Geometry: final body of the model. Coordinates: model frame, mm. A direction names the side the tool comes from. Give positions to 0.01 mm unless a question says otherwise; leave off trailing zeros. Order: outer loops, then holes, each group sorted by start corner. A loop starts at its lowest first (then second) coordinate and runs counter-clockwise, first axis right, second up. Notation, with made-up numbers: (-24, 37) - (-18, 37) arc R34 ccw to (-18, 75) - close; hole circle Ø2 at (-38.75, 55). An arc over 180 degrees is marked (long way). Use one line per item in the form item = value.
from build123d import *

# Parameters (mm, degrees)
ESQUISSE1_W                                    = 138
ESQUISSE1_H                                    = 77
BOSS_EXTRU_1_DEPTH                             = 3
ESQUISSE2_W                                    = 15
ESQUISSE2_H                                    = 77
BOSS_EXTRU_2_DEPTH                             = 30
CONG_1_R                                       = 13.85
ESQUISSE3_W                                    = 138
ESQUISSE3_H                                    = 33
BOSS_EXTRU_3_DEPTH                             = 5
ENL_V_MAT_EXTRU_13_REACH                       = 168.439
ESQUISSE26_W                                   = 15
ESQUISSE26_H                                   = 33
CONG_5_R                                       = 1
ESQUISSE33_W                                   = 11
ESQUISSE33_H                                   = 83.5
ENL_V_MAT_EXTRU_15_DEPTH                       = 28
ESQUISSE34_W                                   = 3.5
ESQUISSE34_H                                   = 33
BOSS_EXTRU_8_DEPTH                             = 25
BOSS_EXTRU_11_DEPTH                            = 33
ESQUISSE35_R                                   = 1
ESQUISSE35_W                                   = 23
ESQUISSE35_H                                   = 14.5
ENL_V_MAT_EXTRU_16_DEPTH                       = 7
ESQUISSE36_W                                   = 7
ESQUISSE36_H                                   = 11.75
ENL_V_MAT_EXTRU_17_DEPTH                       = 2
ESQUISSE44_R                                   = 6
ENL_V_MAT_EXTRU_19_DEPTH                       = 3.5
D_GAGEMENT_M124_D                              = 13.5
D_GAGEMENT_M124_DEPTH                          = 3.5
D_GAGEMENT_M124_TIP                            = 4.055809178
ESQUISSE48_R                                   = 1.5
ENL_V_MAT_EXTRU_20_DEPTH                       = 5
FRAISAGE_POUR_VIS_T_TE_FRAIS_E_M32_D           = 3.4
FRAISAGE_POUR_VIS_T_TE_FRAIS_E_M32_DEPTH       = 5
FRAISAGE_POUR_VIS_T_TE_FRAIS_E_M32_CSINK_D     = 6.3
FRAISAGE_POUR_VIS_T_TE_FRAIS_E_M32_CSINK_ANGLE = 90
FRAISAGE_POUR_VIS_T_TE_FRAIS_E_M32_TIP         = 1.021463052
ESQUISSE52_W                                   = 10
ESQUISSE52_H                                   = 10
BOSS_EXTRU_12_DEPTH                            = 7
ESQUISSE53_R                                   = 1.5
ENL_V_MAT_EXTRU_21_DEPTH                       = 7
CONG_8_R                                       = 5


with BuildPart() as part:
    # Esquisse1 → Boss.-Extru.1 (new body)
    with BuildSketch(Plane(origin=(0, 0, 0), x_dir=(1, 0, 0), z_dir=(0, 1, 0))):
        with Locations((69, 38.5)):
            Rectangle(ESQUISSE1_W, ESQUISSE1_H)
    extrude(amount=BOSS_EXTRU_1_DEPTH)

    # Esquisse2 → Boss.-Extru.2 (add)
    with BuildSketch(Plane(origin=(0, 3, 0), x_dir=(1, 0, 0), z_dir=(0, 1, 0))):
        with Locations((130.5, 38.5)):
            Rectangle(ESQUISSE2_W, ESQUISSE2_H)
    extrude(amount=BOSS_EXTRU_2_DEPTH)

    # Congé1
    cong_1_edges = [part.edges().sort_by_distance(p)[0] for p in [
        (123, 3, -38.5),
    ]]
    fillet(cong_1_edges, radius=CONG_1_R)

    # Esquisse3 → Boss.-Extru.3 (add)
    with BuildSketch(Plane(origin=(0, 0, -77), x_dir=(-1, 0, 0), z_dir=(0, 0, -1))):
        with Locations((-69, 16.5)):
            Rectangle(ESQUISSE3_W, ESQUISSE3_H)
    boss_extru_3 = extrude(amount=BOSS_EXTRU_3_DEPTH)

    # Symétrie1: Boss.-Extru.3 across plane
    add(boss_extru_3.mirror(Plane.XY.offset(-38.5)))

    # Enlèv. mat.-Extru.13: up to this face of the body (flat: up to its plane)
    enl_v_mat_extru_13_end = Plane(part.part.faces().sort_by_distance((69, 16.5, -82))[0])
    # Esquisse26 → Enlèv. mat.-Extru.13 (cut, up to the picked face)
    with BuildSketch(Plane.XY.offset(5), mode=Mode.PRIVATE) as enl_v_mat_extru_13_sk1:
        with Locations((7.5, 16.5)):
            Rectangle(ESQUISSE26_W, ESQUISSE26_H)
    enl_v_mat_extru_13_tool1 = split(extrude(enl_v_mat_extru_13_sk1.sketch, amount=-ENL_V_MAT_EXTRU_13_REACH, mode=Mode.PRIVATE), bisect_by=enl_v_mat_extru_13_end, keep=Keep.BOTH, mode=Mode.PRIVATE)
    add(enl_v_mat_extru_13_tool1.solids().sort_by(Axis((7.5, 16.5, 5), (0, 0, -1)))[0], mode=Mode.SUBTRACT)

    # Congé5
    cong_5_edges = [part.edges().sort_by_distance(p)[0] for p in [
        (123, 24.925, -77),
        (123, 24.925, 0),
        (62.075, 3, -77),
        (118.943428919, 7.056571081, 0),
        (118.943428919, 7.056571081, -77),
        (62.075, 3, 0),
    ]]
    fillet(cong_5_edges, radius=CONG_5_R)

    # Esquisse33 → Enlèv. mat.-Extru.15 (cut)
    with BuildSketch(Plane(origin=(0, 33, 0), x_dir=(1, 0, 0), z_dir=(0, 1, 0))):
        with Locations((132.5, 40.25)):
            Rectangle(ESQUISSE33_W, ESQUISSE33_H)
    extrude(amount=-ENL_V_MAT_EXTRU_15_DEPTH, mode=Mode.SUBTRACT)

    # Esquisse34 → Boss.-Extru.8 (add)
    with BuildSketch(Plane(origin=(138, 0, 0), x_dir=(0, 0, -1), z_dir=(1, 0, 0))):
        with Locations((-3.25, 16.5)):
            Rectangle(ESQUISSE34_W, ESQUISSE34_H)
    extrude(amount=BOSS_EXTRU_8_DEPTH)

    # Esquisse43 → Boss.-Extru.11 (add)
    with BuildSketch(Plane.XZ):
        Polygon((54.5, 5), (58.5, 5), (58.5, 18), (94.5, 18), (94.5, 25), (54.5, 25), align=None)
    extrude(amount=-BOSS_EXTRU_11_DEPTH)

    # Esquisse35 → Enlèv. mat.-Extru.16 (cut)
    with BuildSketch(Plane.XY.offset(25)):
        with Locations((91.8, 19)):
            Circle(ESQUISSE35_R)
        with Locations((64.2, 19)):
            Circle(ESQUISSE35_R)
        with Locations((78, 19)):
            Rectangle(ESQUISSE35_W, ESQUISSE35_H)
    extrude(amount=-ENL_V_MAT_EXTRU_16_DEPTH, mode=Mode.SUBTRACT)

    # Esquisse36 → Enlèv. mat.-Extru.17 (cut)
    with BuildSketch(Plane(origin=(0, 0, 18), x_dir=(-1, 0, 0), z_dir=(0, 0, -1))):
        with Locations((-78, 5.875)):
            Rectangle(ESQUISSE36_W, ESQUISSE36_H)
    extrude(amount=-ENL_V_MAT_EXTRU_17_DEPTH, mode=Mode.SUBTRACT)

    # Esquisse44 → Enlèv. mat.-Extru.19 (cut)
    with BuildSketch(Plane.XY.offset(5)):
        with Locations((147, 19)):
            Circle(ESQUISSE44_R)
    extrude(amount=-ENL_V_MAT_EXTRU_19_DEPTH, mode=Mode.SUBTRACT)

    # Dégagement M124
    with Locations(Plane.XY.offset(5)):
        with Locations((147, 19)):
            Hole(D_GAGEMENT_M124_D / 2, depth=D_GAGEMENT_M124_DEPTH)
            with Locations((0, 0, -(D_GAGEMENT_M124_DEPTH + D_GAGEMENT_M124_TIP / 2))):  # 118° drill point
                Cone(0, D_GAGEMENT_M124_D / 2, D_GAGEMENT_M124_TIP, mode=Mode.SUBTRACT)

    # Esquisse48 → Enlèv. mat.-Extru.20 (cut)
    with BuildSketch(Plane(origin=(0, 5, 0), x_dir=(1, 0, 0), z_dir=(0, 1, 0))):
        with Locations(Location((133, 8.5, 0), (0, 0, 270))):
            Circle(ESQUISSE48_R)
        with Locations(Location((133, 72, 0), (0, 0, 270))):
            Circle(ESQUISSE48_R)
    extrude(amount=-ENL_V_MAT_EXTRU_20_DEPTH, mode=Mode.SUBTRACT)

    # Fraisage pour vis à tête fraisée M32
    with Locations(Plane(origin=(0, 5, 0), x_dir=(1, 0, 0), z_dir=(0, 1, 0))):
        with Locations((133, 72), (133, 8.5)):
            CounterSinkHole(FRAISAGE_POUR_VIS_T_TE_FRAIS_E_M32_D / 2, FRAISAGE_POUR_VIS_T_TE_FRAIS_E_M32_CSINK_D / 2, depth=FRAISAGE_POUR_VIS_T_TE_FRAIS_E_M32_DEPTH, counter_sink_angle=FRAISAGE_POUR_VIS_T_TE_FRAIS_E_M32_CSINK_ANGLE)
            with Locations((0, 0, -(FRAISAGE_POUR_VIS_T_TE_FRAIS_E_M32_DEPTH + FRAISAGE_POUR_VIS_T_TE_FRAIS_E_M32_TIP / 2))):  # 118° drill point
                Cone(0, FRAISAGE_POUR_VIS_T_TE_FRAIS_E_M32_D / 2, FRAISAGE_POUR_VIS_T_TE_FRAIS_E_M32_TIP, mode=Mode.SUBTRACT)

    # Esquisse52 → Boss.-Extru.12 (add)
    with BuildSketch(Plane.XZ):
        with Locations((20, 10)):
            Rectangle(ESQUISSE52_W, ESQUISSE52_H)
    boss_extru_12 = extrude(amount=-BOSS_EXTRU_12_DEPTH)

    # Esquisse53 → Enlèv. mat.-Extru.21 (cut)
    with BuildSketch(Plane(origin=(0, 7, 0), x_dir=(1, 0, 0), z_dir=(0, 1, 0))):
        with Locations(Location((20, -10, 0), (0, 0, 270))):
            Circle(ESQUISSE53_R)
    enl_v_mat_extru_21 = extrude(amount=-ENL_V_MAT_EXTRU_21_DEPTH, mode=Mode.SUBTRACT)

    # Esquisse55 → Fraisage pour vis à tête fraisée M33 (revolve, cut)
    with BuildSketch(Plane(origin=(20, 7, 10), x_dir=(0, 0, 1), z_dir=(1, 0, 0))):
        Polygon((0, 0), (0, 8.021463052), (1.7, 7), (1.7, 1.45), (3.15, 0), align=None)
    fraisage_pour_vis_t_te_frais_e_m33 = revolve(axis=Axis((20, 13.35, 10), (0, -1, 0)), mode=Mode.SUBTRACT)

    # Symétrie2: Boss.-Extru.12, Enlèv. mat.-Extru.21, Fraisage pour vis à tête fraisée M33 across plane
    add(boss_extru_12.mirror(Plane.XY.offset(-38.5)))
    add(enl_v_mat_extru_21.mirror(Plane.XY.offset(-38.5)), mode=Mode.SUBTRACT)
    add(fraisage_pour_vis_t_te_frais_e_m33.mirror(Plane.XY.offset(-38.5)), mode=Mode.SUBTRACT)

    # Congé8
    cong_8_edges = [part.edges().sort_by_distance(p)[0] for p in [
        (25, 3.5, 5),
        (25, 3.5, 15),
        (15, 3.5, 15),
        (15, 3.5, -92),
        (25, 3.5, -92),
        (25, 3.5, -82),
    ]]
    fillet(cong_8_edges, radius=CONG_8_R - 0.0001)  # a hair under: the kernel refuses the full size


solid = part.part
(1) Cut plane A-A on z = -72. Output: boundary loops of the cut face in (x, y).
Computed values:
outline = (15, 0) - (131.3, 0) - (131.3, 3.55) - (129.85, 5) - (127, 5) - (127, 33) - (123, 33) - (123, 16.85) arc R13.85 cw to (109.15, 3) - (15, 3) - close; (134.7, 0) - (138, 0) - (138, 5) - (136.15, 5) - (134.7, 3.55) - close
(2) Ray query, line 1 along Z through (x, y) = (20, 2.6); line 2 along Z through (x, y) = (92, 30); line 3 along Z through (x, y) = (102.5, 9.5). Return the intervals inside material, ascending.
Computed values:
line_1 = -92 to -88.7, -85.3 to 8.3, 11.7 to 15
line_2 = -82 to -77, 0 to 5, 18 to 25
line_3 = -82 to -77, 0 to 5
(3) Cut plane B-B on x = 147. Output: boundary loops of the cut face in (y, z).
Computed values:
outline = (0, 1.5) - (12.25, 1.5) - (12.25, 5) - (0, 5) - close; (25.75, 1.5) - (33, 1.5) - (33, 5) - (25.75, 5) - close
(4) Contact query for flat-ended pins moving along their axis: pin 1 Ø5 at (y, z) = (23, -47.5) entering from -X; pin 2 Ø8.5 at (x, y) = (46.5, 24.5) entering from -Z; pin 3 Ø3.5 at (y, z) = (18.5, 20.5) entering from +X. Output: stop coordinate, or through.
Computed values:
pin_1 = 123
pin_2 = -82
pin_3 = 94.5
(5) Cut plane C-C on x = 32. Output: boundary loops of the cut face in (y, z), plus the area to 3 significant figures.
Computed values:
outline = (0, -82) - (33, -82) - (33, -77) - (4, -77) arc R1 cw to (3, -76) - (3, -1) arc R1 cw to (4, 0) - (33, 0) - (33, 5) - (0, 5) - close
area = 561 mm²
(6) Cut plane D-D on z = -41. Output: boundary loops of the cut face in (x, y).
Computed values:
outline = (15, 0) - (138, 0) - (138, 5) - (127, 5) - (127, 33) - (123, 33) - (123, 16.85) arc R13.85 cw to (109.15, 3) - (15, 3) - close
(7) Pull-direction query (Z, two-part tool) for faces 1 (the face through (110, 16, 5)), 2 (the face through (75, 9, 25)), 3 (the face through (140.765, 16.415, 3.226)); classes: released by +Z, released by -Z, zero draft, split by the parting line, or undercut.
Computed values:
face_1 = undercut
face_2 = released by +Z
face_3 = zero draft
(8) Reachability of faces 4 (the face through (34, 16, 5)), 5 (the face through (89.5, 19, 22)), 6 (the face through (78, 6, 20)) from +Z, -Z, +X, -X, +Y, -Y: full face, straight path, thin tool, end or side. Return the list, or none.
Computed values:
face_4 = +Z, +Y
face_5 = +Z
face_6 = -Y
